from build123d import *

# Parameters (mm, degrees)
SALIENTE_EXTRUIR1_DEPTH = 2
CROQUIS2_R              = 1.5
CORTAR_EXTRUIR2_DEPTH   = 3
CROQUIS4_R              = 1.5
SALIENTE_EXTRUIR3_DEPTH = 5


with BuildPart() as part:
    # Croquis1 → Saliente-Extruir1 (new body)
    with BuildSketch(Plane(origin=(0, 0, 0), x_dir=(1, 0, 0), z_dir=(0, 1, 0))):
        with BuildLine():
            add(Edge.make_bspline(
                [(-0.047552943, -5.41433386), (1.239779979, -3.635052884), (2.414610314, -1.780353063)],
                knots=[0, 0, 0, 1, 1, 1], degree=2))
            ThreePointArc((2.414610314, -1.780353063), (1.832628676, 2.375178338), (-2.334614821, 1.88403122))
            add(Edge.make_bspline(
                [(-2.334614821, 1.88403122), (-2.951325259, 1.119828741), (-4.509299118, -0.563300275), (-5.988366098, -3.121312175), (-9.777324233, -3.72498405), (-12.108475468, -3.349116626), (-13.205411179, -2.56941452)],
                knots=[0, 0, 0, 0, 0.210355785, 0.457410568, 0.578047142, 0.870899615, 0.870899615, 0.870899615, 0.870899615], degree=3))
            add(Edge.make_bspline(
                [(-13.205411179, -2.56941452), (-15.819352109, -0.83375271), (-17.897343033, 1.511058614)],
                knots=[0, 0, 0, 1, 1, 1], degree=2))
            ThreePointArc((-17.897343033, 1.511058614), (-21.528082135, 2.135894472), (-21.839041513, -1.535071415))
            add(Edge.make_bspline(
                [(-18.257712787, -4.881966223), (-20.206095591, -3.376965901), (-21.839041513, -1.535071415)],
                knots=[0, 0, 0, 1, 1, 1], degree=2))
            add(Edge.make_bspline(
                [(-13.205411179, -7.886532608), (-14.054265837, -7.471831244), (-15.806738264, -6.580922778), (-17.428856772, -5.469594286), (-18.257712787, -4.881966223)],
                knots=[0, 0, 0, 0, 0.481848673, 1, 1, 1, 1], degree=3))
            add(Edge.make_bspline(
                [(-9.554936668, -9.109021082), (-11.480606525, -8.82957168), (-13.205411179, -7.886532608)],
                knots=[0, 0, 0, 1, 1, 1], degree=2))
            add(Edge.make_bspline(
                [(-0.047552943, -5.41433386), (-1.436995415, -7.008044472), (-4.467557841, -9.495004111), (-8.188902662, -9.306395591), (-9.554936668, -9.109021082)],
                knots=[0, 0, 0, 0, 0.608220397, 1, 1, 1, 1], degree=3))
        make_face()
    extrude(amount=SALIENTE_EXTRUIR1_DEPTH)

    # Croquis2 → Cortar-Extruir2 (cut)
    with BuildSketch(Plane(origin=(0, 2, 0), x_dir=(1, 0, 0), z_dir=(0, 1, 0))):
        Circle(CROQUIS2_R)
    extrude(amount=-CORTAR_EXTRUIR2_DEPTH, mode=Mode.SUBTRACT)

    # Croquis4 → Saliente-Extruir3 (add)
    with BuildSketch(Plane(origin=(0, 2, 0), x_dir=(1, 0, 0), z_dir=(0, 1, 0))):
        with Locations((-19.999377879, 0.157748042)):
            Circle(CROQUIS4_R)
    extrude(amount=SALIENTE_EXTRUIR3_DEPTH)


solid = part.part
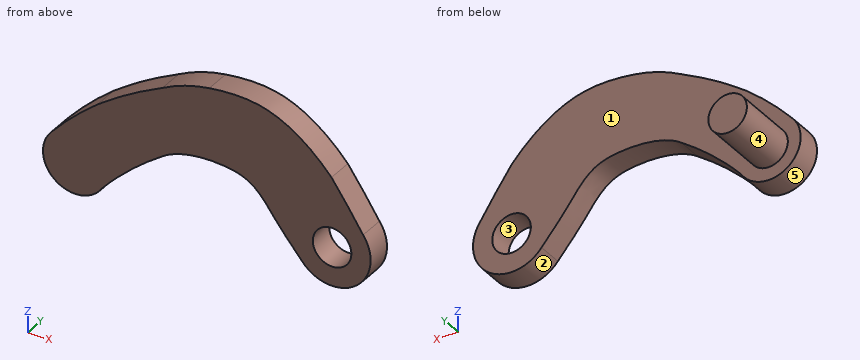
Work out the finished part from the listing and answer in its coordinate system (mm). Face numbers are marked on the shaded views. A direction names the side the tool comes from. Give positions to 0.01 mm unless a question says otherwise; leave off trailing zeros. Order: outer loops, then holes, each group sorted by start corner. A loop starts at its lowest first (then second) coordinate and runs counter-clockwise, first axis right, second up. Notation, with made-up numbers: (68, 32) -> (73, 32) arc R33 ccw to (73, 60) -> close; hole circle Ø7 at (-38, 82). An arc over 180 degrees is marked (long way). One line per item, written item: value.
Item 1: Find section A-A, the plane y = 5.5. Give the vertices of the cut face in (x, z), plus the area to 3 significant figures.
Answer sheet:
outline: circle Ø3 at (-20, -0.16)
area: 7.07 mm²
Item 2: Flat-ended cylindrical pins translate along their axes: P1, Ø4, axis at x = -2, y = 2, coming from the +Z side; P2, Ø3, axis at y = 1.5, z = 7.5, coming from the +X side; P3, Ø3.5, axis at x = -8, z = 1.5, coming from the +Y side. Find the tip coordinate at first contact, or state that the pin passes through.
Answer sheet:
P1: z = 8.55
P2: x = -0.58
P3: through
Item 3: A tool of negligible diameter and unlimited length cuts with its end or side. For the marked faces 4 and 5, from which of +Z, -Z, +X, -X, +Y, -Y can it reach the whole face along a straight path? Write none if from no direction.
Answer sheet:
face 4: +Y
face 5: +Y, -Y
Item 4: Determine the mould class of the marked faces 1, 2 and 3 for opening direction Z: released by +Z, released by -Z, zero draft, split by the parting line, or undercut.
Answer sheet:
face 1: zero draft
face 2: split by the parting line
face 3: undercut
Item 5: Straight lines are drawn through the part: probe 1 along X at (y, z) = (0.5, 0); probe 2 along X at (y, z) = (1.25, 0.25); probe 3 along Y at (x, z) = (-13.5, 3). For each, find the intervals that lie inside material, in ascending order.
Answer sheet:
probe 1: -22.49 to -16.44, -3.91 to -1.5, 1.5 to 3
probe 2: -22.47 to -16.17, -4.11 to -1.48, 1.48 to 2.99
probe 3: 0 to 2
